Verification items for the finished model (mm, model axes). A direction names the side the tool comes from. Give positions to 0.01 mm unless a question says otherwise; leave off trailing zeros. Order: outer loops, then holes, each group sorted by start corner. A loop starts at its lowest first (then second) coordinate and runs counter-clockwise, first axis right, second up.
(1) Gauge pin test, flat ends, axial feed: pin 1 (3 mm diameter, centred on y = 16.5, z = 13, fed in from -X); pin 2 (5 mm diameter, centred on x = 6, y = -15.5, fed in from +Z); pin 3 (2 mm diameter, centred on x = 17.5, z = 51, fed in from -Y); pin 4 (8 mm diameter, centred on x = 25.5, z = 15.5, fed in from +Y). Record the tip position at first contact, or that the pin passes through.
(2) Mould release check, pull along X, two halves, no side actions. Record for faces 3 (the face through (-43.54, -9.87, 37.57)), 4 (the face through (-5.883, -14.419, 49.528)): pulls with the +X half, pulls with the -X half, needs draft (parallel to the pull), parting line crosses it, or undercut.
(3) Sectioned sample at A-A on y = 6.5. Count the separate pieces of the cut face and the enclosed holes in it, plus the area to 3 significant figures.
(4) Access from +Z, -Z, +X, -X, +Y, -Y to the whole of each face (thin tool, end or side, straight path). Record for faces 1 (the face through (63.648, 31.088, 49.528)), 2 (the face through (43.75, 31.44, 37.57)).
(5) Sectioned sample at C-C on z = 11. Record the cut outline in (x, y).
(6) Scan lines: L1, parallel to X at y = -24.5, z = 13; L2, parallel to Y at x = 39, z = 15; L3, parallel to X at y = -18, z = 9. Record each from-to range of solid material in increasing order.
(7) Sectioned sample at B-B on x = -53.5. Record the cut outline in (y, z).
```python
from build123d import *

# Parameters (mm, degrees)
F1_DEPTH = 76.2
F3_DEPTH = 54.102


with BuildPart() as f1:
    # F0 (on Top) → F1 (new body)
    with BuildSketch(Plane.XY):
        Polygon((-48.208792, 53.739436), (-43.231208, 15.209274), (-67.934759, 49.314924), (-31.875403, -7.264898), (-65.353796, 9.125564), (-21.108629, -29.404595), (-2.911252, 3.61714), (-13.365726, -40.465888), (-60.007501, -29.404595), (0, -52.633308), (50.870309, -3.450001), (29.588953, -46.918306), (55.398632, -69.040887), (45.627821, -42.49379), (72.359271, 17.974596), (60.929276, 38.622338), (26.086211, 24.058307), (63.510239, 24.058307), (5.622822, -25.164437), (8.572499, 63.141532), (-8.756855, 27.745403), (-16.131049, 69.040887), (-16.131049, -13.734437), align=None)
    extrude(amount=F1_DEPTH)

    # F2 (on face) → F3 (cut)
    with BuildSketch(Plane.XY.offset(76.2)):
        Polygon((-14.861049, 54.704386), (-14.861049, -15.436109), (0.475501, 12.394247), (-12.423058, -41.994671), (-42.220324, -34.928124), (-0.2989, -51.155774), (55.197442, 2.500153), (31.161853, -46.593818), (52.522279, -64.902753), (44.258507, -42.450249), (70.942717, 17.911278), (66.877654, 25.254621), (4.257654, -27.992326), (7.105206, 57.256262), (-9.324238, 23.698248), align=None)
        Polygon((60.369236, 37.011767), (32.417664, 25.328307), (66.836864, 25.328307), align=None)
        Polygon((-41.332285, 10.422641), (-43.910667, 13.982347), (-28.376483, -10.391947), (-57.22765, 3.733103), (-21.461381, -27.413352), (-15.863477, -17.255159), (-45.925721, 45.979215), align=None)
    extrude(amount=-F3_DEPTH, mode=Mode.SUBTRACT)


solid = f1.part
```
Ans:
1. pin 1: stops at x = -47.98
1. pin 2: stops at z = 76.2
1. pin 3: stops at y = -36.68
1. pin 4: stops at y = 25.49
2. face 3: pulls with the -X half
2. face 4: undercut
3. separate pieces: 4
3. enclosed holes: 0
3. area: 2,130 mm2
4. face 1: +Z
4. face 2: +Z, -Z, +Y
5. outline: (-67.93, 49.31) - (-31.88, -7.26) - (-65.35, 9.13) - (-21.11, -29.4) - (-2.91, 3.62) - (-13.37, -40.47) - (-60.01, -29.4) - (0, -52.63) - (50.87, -3.45) - (29.59, -46.92) - (55.4, -69.04) - (45.63, -42.49) - (72.36, 17.97) - (60.93, 38.62) - (26.09, 24.06) - (63.51, 24.06) - (5.62, -25.16) - (8.57, 63.14) - (-8.76, 27.75) - (-16.13, 69.04) - (-16.13, -13.73) - (-48.21, 53.74) - (-43.23, 15.21) - close
6. L1: x = -26.74 to -18.41, -9.58 to 5.65, 6.4 to 29.1, 40.56 to 53.58
6. L2: y = -54.98 to -27.7, -14.93 to 3.22, 24.06 to 29.46
6. L3: x = -34.2 to -14.82, -8.04 to 5.86, 14.05 to 35.82, 43.75 to 56.46
7. outline: (-31.92, 0) - (-30.95, 0) - (-30.95, 76.2) - (-31.92, 76.2) - close; (-1.2, 0) - (3.32, 0) - (3.32, 76.2) - (1.91, 76.2) - (1.91, 22.1) - (0.49, 22.1) - (0.49, 76.2) - (-1.2, 76.2) - close; (26.67, 0) - (29.39, 0) - (29.39, 76.2) - (26.67, 76.2) - close
